Drawing for the job (mm, zero at the part's lowest x, y, z). Give positions to 0.01 mm unless a question says otherwise; leave off trailing zeros. Write each loop counter-clockwise with the first axis right and the second up, starting at its lowest first coordinate (ties: lowest second). Pieces come first, ordered by that corner, then holes. Notation, with made-up numbers: M -25,-5 L -20,-5 A24 ccw -20,32 Z; hole C 19.25,71.25 d3. An arc over 180 degrees is marked long. Write item = value, one per line. Start each with the question number.
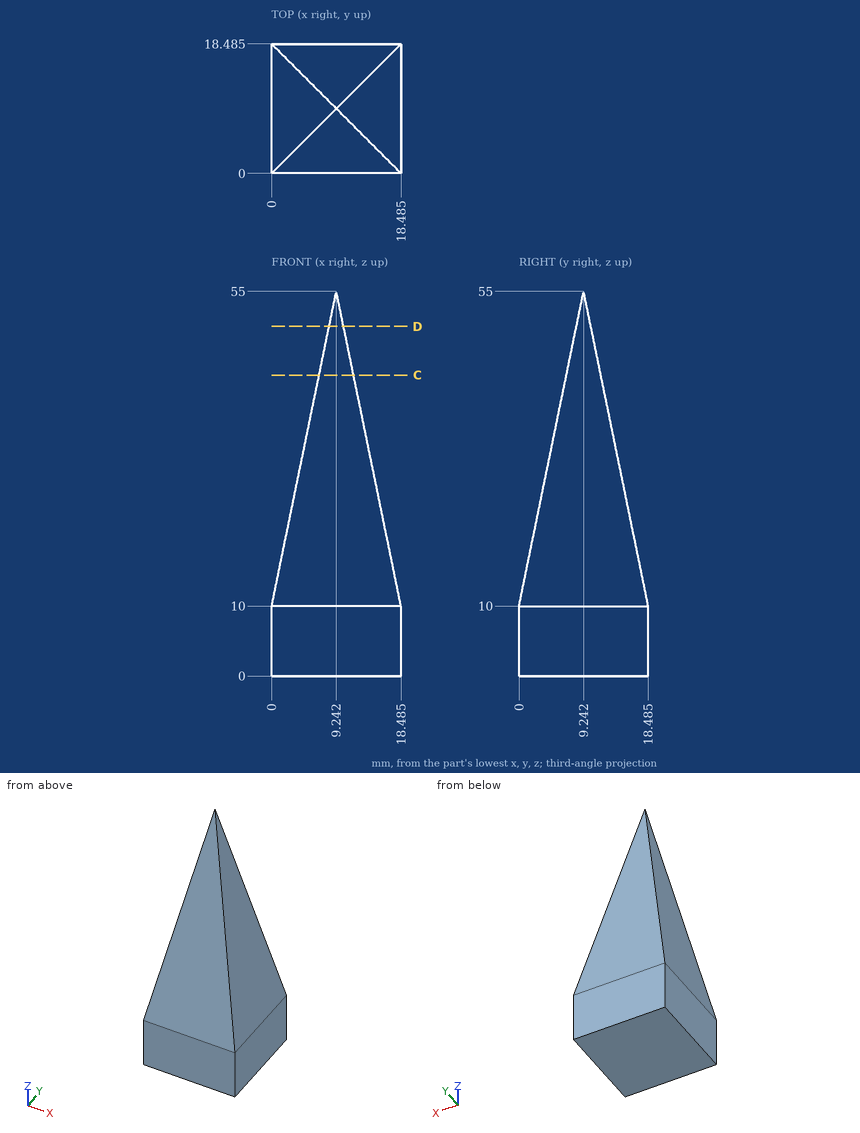
Q1. Drop flat-ended pins along their axis: P1, Ø5, axis at x = 9, z = 26, coming from the +Y side; P2, Ø1.5, axis at x = 4, y = 15, coming from the -Z side. Give the stop position or say it passes through.
Q2. Probe line 1 along Y through (x, z) = (8.5, 24) (1 decimal); line 2 along X through (y, z) = (11.5, 40); line 3 along Y through (x, z) = (5.25, 26.5) (1 decimal). List the from-to ranges inside material, lowest first.
Q3. Slice it at D-D (z = 50). Give the cut face in (x, y) (1 decimal).
Q4. Slice it at C-C (z = 43). Give the cut face in (x, y).
Working result:
q1.P1 = 15.71
q1.P2 = 0
q2.line_1 = 2.9 to 15.6
q2.line_2 = 6.16 to 12.32
q2.line_3 = 3.4 to 15.1
q3.outline = M 8.2,8.2 L 10.3,8.2 L 10.3,10.3 L 8.2,10.3 Z
q4.outline = M 6.78,6.78 L 11.71,6.78 L 11.71,11.71 L 6.78,11.71 Z
